```python
from build123d import *

# Parameters (mm, degrees)
SKETCH_W        = 27
SKETCH_H        = 38
PAD_DEPTH       = 45
POCKET_DEPTH    = 38.001
POCKET001_DEPTH = 36
POCKET002_DEPTH = 27.001
PAD001_DEPTH    = 1
PAD002_DEPTH    = 1
SKETCH008_W     = 27
SKETCH008_H     = 22
PAD003_DEPTH    = 1
SKETCH009_R     = 1.75
POCKET003_DEPTH = 45.002679


with BuildPart() as part:
    # Sketch → Pad (new body)
    with BuildSketch(Plane.XY):
        with Locations((-29.5, -13)):
            Rectangle(SKETCH_W, SKETCH_H)
    extrude(amount=-PAD_DEPTH)

    # Sketch003 (on Face2 of Pad) → Pocket (cut, through all)
    with BuildSketch(Plane.XZ.offset(32)):
        with BuildLine():
            ThreePointArc((-44, 0), (-34.593948, -26.908525), (-14.407019, -47.033892))
            Line((-14.407019, -47.033892), (-67.061646, -46.193626))
            Line((-67.061646, -46.193626), (-44, 0))
        make_face()
    extrude(amount=-POCKET_DEPTH, mode=Mode.SUBTRACT)

    # Sketch004 (on Face3 of Pocket) → Pocket001 (cut)
    with BuildSketch(Plane.XZ.offset(32)):
        with BuildLine():
            ThreePointArc((-29, 0), (-23.639101, -24.573945), (-8.645898, -44.768545))
            Line((-8.645898, -44.768545), (-11.371384, -46.875244))
            ThreePointArc((-42, 0), (-32.20336, -27.042905), (-11.371384, -46.875244))
            Line((-29, 0), (-42, 0))
        make_face()
    extrude(amount=-POCKET001_DEPTH, mode=Mode.SUBTRACT)

    # Sketch005 (on Face1 of Pocket001) → Pocket002 (cut, through all)
    with BuildSketch(Plane.YZ.offset(-16)):
        Polygon((15.686372, 17.350435), (-17.648283, -56.610836), (15.686372, -59.996391), align=None)
    extrude(amount=-POCKET002_DEPTH, mode=Mode.SUBTRACT)

    # Sketch006 (on Face3 of Pocket002) → Pad001 (join)
    with BuildSketch(Plane.XZ.offset(32)):
        with BuildLine():
            ThreePointArc((-43, -6.191343), (-33.888802, -28.004267), (-17.459999, -45.001679))
            Line((-17.459999, -45.001679), (-16, -45))
            Line((-16, 0), (-16, -45))
            Line((-43, 0), (-16, 0))
            Line((-43, -6.191343), (-43, 0))
        make_face()
    extrude(amount=-PAD001_DEPTH)

    # Sketch007 (on Face5 of Pad001) → Pad002 (join)
    with BuildSketch(Plane(origin=(0, 6.538304, -2.946841), x_dir=(-1, 0, 0), z_dir=(0, 0.911681, -0.410898))):
        with BuildLine():
            Line((16, -1.310067), (43, -1.310067))
            ThreePointArc((17.46237, -46.127049), (34.375924, -26.080314), (43, -1.310067))
            Line((16, -46.127049), (17.46237, -46.127049))
            Line((16, -1.310067), (16, -46.127049))
        make_face()
    extrude(amount=-PAD002_DEPTH)

    # Sketch008 (on Face2 of Pad002) → Pad003 (join)
    with BuildSketch(Plane.XY):
        with Locations((-29.5, -21)):
            Rectangle(SKETCH008_W, SKETCH008_H)
    extrude(amount=-PAD003_DEPTH)

    # Sketch009 (on Face2 of Pad003) → Pocket003 (cut, through all)
    with BuildSketch(Plane.XY):
        with Locations((-23.410666, -26)):
            Circle(SKETCH009_R)
    extrude(amount=-POCKET003_DEPTH, mode=Mode.SUBTRACT)


solid = part.part
```
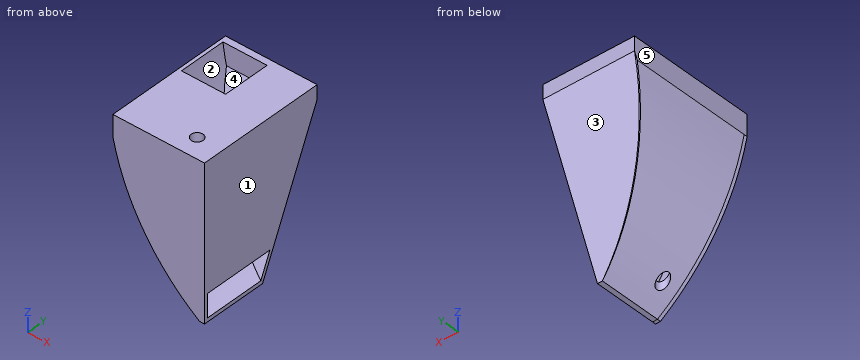
The model under review builds one solid part; all positions refer to its coordinate system, in mm. Face numbers are marked on the shaded views. A direction names the side the tool comes from. Give positions to 0.01 mm unless a question says otherwise; leave off trailing zeros. Loops run counter-clockwise (first coordinate to the right, second up) from the corner with the lowest first, then second, coordinate; pieces in that order, holes last. Notation, with made-up numbers: (15, 40) - (19, 40) arc R16 ccw to (19, 53) - close; hole circle Ø3 at (-3, -17). An arc over 180 degrees is marked (long way). Answer as a JSON object with one key per item and string values.
Q1. Mouldability with a two-part tool opening along X and no side actions: class the marked faces 1, 2 and 3 as +X half, -X half, draft (parallel to the pull), parting line (faces both ways), or undercut.
Worked out:
{"face 1": "+X half", "face 2": "undercut", "face 3": "draft"}
Q2. Insertion check: pin 1 (14 mm diameter, centred on x = -35.5, y = -16.5, fed in from -Z); pin 2 (5.5 mm diameter, centred on x = -23.41, y = -26, fed in from -Z); pin 3 (12 mm diameter, centred on x = -27, z = -23.5, fed in from +Y). Each pin has a flat end and moves straight along its axis. Give the tip position at first contact, or say it passes through.
Worked out:
{"pin 1": "stops at z = -35.07", "pin 2": "stops at z = -42.58", "pin 3": "stops at y = -0.02"}
Q3. To check wall thickness, follow line 1 along X through (y, z) = (-26, -13.25); line 2 along X through (y, z) = (-26, -18.25); line 3 along X through (y, z) = (-27.5, -39). State the ranges of each line that lie inside material, in increasing order.
Worked out:
{"line 1": "x = -41.07 to -38.97, -27.47 to -25.16, -21.66 to -16", "line 2": "x = -39.15 to -36.99, -26.09 to -25.16, -21.66 to -16", "line 3": "x = -24.73 to -24.31, -22.51 to -22.05"}
Q4. For the marked faces 4 and 5, list the 3-axis set-ups (+Z, -Z, +X, -X, +Y, -Y) from which the entire face can be reached by the end or side of a thin tool; tool diameter is ignored.
Worked out:
{"face 4": "none", "face 5": "+Z, -Z, -X, +Y, -Y"}
Q5. Add section A-A on y = -26. State the section outline as (x, z) points.
Worked out:
{"outline": "(-43, -6.19) arc R63.79 ccw to (-25.16, -38.59) - (-25.16, -35.94) arc R62.76 cw to (-41.87, -1) - (-28.99, -1) arc R59.79 ccw to (-25.16, -20.91) - (-25.16, 0) - (-43, 0) - close; (-21.66, -41.76) arc R63.79 ccw to (-17.46, -45) - (-16, -45) - (-16, -43.89) arc R62.76 cw to (-21.66, -39.35) - close; (-21.66, -28.53) arc R59.79 ccw to (-16, -37.05) - (-16, 0) - (-21.66, 0) - close"}
